For this review, take the finished solid that the model builds, in its own axes (mm). Face numbers are marked on the shaded views. A direction names the side the tool comes from. Coordinates: 2 decimals unless noted, no trailing zeros. Loops run counter-clockwise (first coordinate to the right, second up) from the corner with the lowest first, then second, coordinate; pieces in that order, holes last. Notation, with made-up numbers: (80.25, -7.75) - (104.25, -7.75) arc R37 ccw to (104.25, 28.25) - close; hole circle Ø3 at (-30, 13). An arc over 180 degrees is marked (long way). One line per item, written item: value. Start each with the question number.
1. Take a section at D-D, the plane z = 13.5. State the section outline as (x, y) points, and give its area (3 significant figures).
2. To check wall thickness, follow line 1 (X direction, y = 33.5, z = 11.5); line 2 (Y direction, x = -11, z = 14.75); line 3 (Z direction, x = -39, y = 28). State the ranges of each line that lie inside material, in increasing order. Write a range as from..to.
3. Take a section at B-B, the plane x = -17. State the section outline as (y, z) points, and give its area (3 significant figures).
4. Take a section at C-C, the plane y = 23. State the section outline as (x, z) points, and give its area (3 significant figures).
5. Insertion check: pin 1 (1.5 mm diameter, centred on y = 24, z = 20, fed in from -X); pin 2 (4 mm diameter, centred on y = 43.5, z = 14.5, fed in from +X); pin 3 (1.8 mm diameter, centred on x = 1.5, z = 12.5, fed in from +Y). Each pin has a flat end and moves straight along its axis. Give the tip position at first contact, or say it passes through.
6. The part is to be moulded in two halves that separate along X. For the marked faces 5, 6, 7 and 8, say which applies: released by +X, released by -X, zero draft, split by the parting line, or undercut.
7. For the marked faces 1, 2, 3 and 4, list the 3-axis set-ups (+Z, -Z, +X, -X, +Y, -Y) from which the entire face can be reached by the end or side of a thin tool; tool diameter is ignored.
8. Take a section at A-A, the plane z = 19.25. State the section outline as (x, y) points.
Autodesk Inventor part; units mm, degrees
ref_plane "Work Plane1" through (0, 0, 10) normal (0, 0, 1) x (1, 0, 0)
ref_plane "Work Plane3" through (-33.4299, 11.4299, 16.4) normal (0, 0, -1) x (0, 1, 0)
ref_plane "YZ Plane" through (0, 0, 0) normal (1, 0, 0) x (0, 1, 0)
ref_plane "Work Plane1" through (0, 0, 10) normal (0, 0, 1) x (1, 0, 0)
sketch "Sketch1" plane through (0, 0, 10) normal (0, 0, 1) x (1, 0, 0)
  line L0 (-4.0299, -0.3538) -> (-2.2322, 1.4439) construction
  arc A0 (-1.4439, 2.2322) -> (-2.2322, 1.4439) centre (-0.9299, 0.9299) ccw construction
  line L1 (-1.4439, 2.2322) -> (0.3538, 4.0299) construction
  line L2 (-37.8299, 42.2137) -> (-37.8299, 45.8299) construction
  line L3 (-37.8299, 45.8299) -> (-4.0299, 45.8299) construction
  line L4 (-4.0299, 45.8299) -> (-4.0299, 42.2137) construction
  line L5 (-4.0299, 4.0299) -> (0.3538, 4.0299)
  circle A1 centre (-20.9299, 20.9299) radius 17.5
  line L6 (-20.9299, 58.9723) -> (17.1124, 20.9299) construction
  line L7 (17.1124, 20.9299) -> (-20.9299, -17.1124) construction
  line L8 (-20.9299, -17.1124) -> (-58.9723, 20.9299) construction
  line L9 (-58.9723, 20.9299) -> (-20.9299, 58.9723) construction
  line L10 (-20.9299, 58.9723) -> (-20.9299, -17.1124) construction
  line L11 (17.1124, 20.9299) -> (-58.9723, 20.9299) construction
  line L12 (-20.9299, 58.9723) -> (32.8701, 58.9723) construction
  line L13 (-43.4299, 43.4299) -> (1.5701, 43.4299) construction
  line L14 (1.5701, 43.4299) -> (1.5701, -1.5701) construction
  line L15 (1.5701, -1.5701) -> (-43.4299, -1.5701) construction
  line L16 (-43.4299, -1.5701) -> (-43.4299, 43.4299) construction
  line L17 (-43.4299, 43.4299) -> (1.5701, -1.5701) construction
  line L18 (1.5701, 43.4299) -> (-43.4299, -1.5701) construction
  line L19 (-43.4299, 5.3876) -> (-43.4299, 36.4723)
  line L20 (-43.4299, 36.4723) -> (-36.4723, 43.4299)
  line L21 (-36.4723, 43.4299) -> (-5.3876, 43.4299)
  line L22 (-5.3876, 43.4299) -> (1.5701, 36.4723)
  line L23 (1.5701, 36.4723) -> (1.5701, 5.3876)
  line L24 (1.5701, 5.3876) -> (-5.3876, -1.5701)
  line L25 (-5.3876, -1.5701) -> (-36.4723, -1.5701)
  line L26 (-36.4723, -1.5701) -> (-43.4299, 5.3876)
  line L27 (-4.0299, 42.2137) -> (-37.8299, 42.2137)
  line L28 (-4.0299, -0.3538) -> (-4.0299, 4.0299)
  circle A2 centre (-20.9299, 20.9299) radius 7.0417
  point P0 (-37.8299, 4.0299)
  dimension "d18" = 53.8
  dimension "d19" = 45
  dimension "d20" = 53.8
  dimension "d21" = 45
  dimension "d22" = 45
extrude "Extrusion1" add sketch "Sketch1" along normal blind 8 contours L28 L24 L25 L26 L19 L20 L27 L22 L23 L5 | L5 L24 L28 | L27 L20 L21 L22 | A1
sketch "Sketch3" plane through (0, 0, 10) normal (0, 0, -1) x (-1, 0, 0)
  line L0 (37.8299, -0.4701) -> (37.8299, 4.0299) construction
  line L1 (4.0299, 4.0299) -> (4.0299, -0.4701) construction
  line L2 (37.8299, -0.4701) -> (37.8299, 1.1886) construction
  line L3 (4.0299, -3.9701) -> (4.0299, -0.3538) construction
  line L4 (45.8299, 4.0299) -> (42.2137, 4.0299) construction
  line L5 (-0.3538, 4.0299) -> (-3.9701, 4.0299) construction
  line L6 (-3.9701, 37.8299) -> (-0.3538, 37.8299) construction
  line L7 (4.0299, 42.2137) -> (4.0299, 45.8299) construction
  line L8 (37.8299, 45.8299) -> (37.8299, 42.2137) construction
  line L9 (42.2137, 37.8299) -> (45.8299, 37.8299) construction
  line L10 (37.8299, 37.7299) -> (45.8299, 37.7299)
  line L11 (45.8299, 37.7299) -> (45.8299, 4.1299)
  line L12 (45.8299, 4.1299) -> (37.8299, 4.1299)
  line L13 (37.8299, 4.1299) -> (37.8299, 37.7299)
  line L14 (37.7299, 4.0299) -> (4.1299, 4.0299)
  line L15 (4.1299, 4.0299) -> (4.1299, -3.9701)
  line L16 (4.1299, -3.9701) -> (37.7299, -3.9701)
  line L17 (37.7299, -3.9701) -> (37.7299, 4.0299)
  line L18 (4.0299, 4.1299) -> (-3.9701, 4.1299)
  line L19 (-3.9701, 4.1299) -> (-3.9701, 37.7299)
  line L20 (-3.9701, 37.7299) -> (4.0299, 37.7299)
  line L21 (4.0299, 37.7299) -> (4.0299, 4.1299)
  line L22 (4.1299, 37.8299) -> (37.7299, 37.8299)
  line L23 (37.7299, 37.8299) -> (37.7299, 45.8299)
  line L24 (37.7299, 45.8299) -> (4.1299, 45.8299)
  line L25 (4.1299, 45.8299) -> (4.1299, 37.8299)
  point P0 (0, 0)
  dimension "d23" = 0.1
  dimension "d24" = 0.1
  dimension "d25" = 0.1
  dimension "d26" = 0.1
  dimension "d27" = 0.1
extrude "Extrusion3" add sketch "Sketch3" against normal up to surface (8 mm away)
sketch "Sketch4" plane through (0, 0, 18) normal (0, 0, 1) x (1, 0, 0)
  line L0 (-33.4299, 35.4299) -> (-33.4299, 11.4299) construction
  line L1 (-33.4299, 11.4299) -> (-8.4299, 11.4299) construction
  line L2 (-8.4299, 11.4299) -> (-8.4299, 35.4299) construction
  line L3 (-8.4299, 35.4299) -> (-33.4299, 35.4299) construction
  circle A0 centre (-10.4299, 33.4299) radius 1.05 construction
  circle A1 centre (-10.4299, 20.9299) radius 1.05 construction
  circle A2 centre (-31.4299, 20.9299) radius 1.05 construction
  circle A3 centre (-31.4299, 33.4299) radius 1.05 construction
  line L4 (-15.4299, 29.8299) -> (-12.4299, 29.8299) construction
  line L5 (-15.4299, 31.8299) -> (-15.4299, 29.8299) construction
  line L6 (-12.4299, 31.8299) -> (-15.4299, 31.8299) construction
  line L7 (-12.4299, 29.8299) -> (-12.4299, 31.8299) construction
  line L8 (-8.4299, 35.4299) -> (-11.9299, 35.4299)
  line L9 (-11.9299, 35.4299) -> (-11.9299, 19.4299)
  line L10 (-11.9299, 19.4299) -> (-8.4299, 19.4299)
  line L11 (-8.4299, 19.4299) -> (-8.4299, 35.4299)
  line L12 (-33.4299, 35.4299) -> (-29.9299, 35.4299)
  line L13 (-29.9299, 35.4299) -> (-29.9299, 19.4299)
  line L14 (-29.9299, 19.4299) -> (-33.4299, 19.4299)
  line L15 (-33.4299, 19.4299) -> (-33.4299, 35.4299)
  line L16 (-33.4299, 35.4299) -> (-37.4299, 35.4299)
  line L17 (-37.4299, 35.4299) -> (-37.4299, 19.4299)
  line L18 (-37.4299, 19.4299) -> (-33.4299, 19.4299)
  line L19 (-33.4299, 19.4299) -> (-33.4299, 35.4299)
  line L20 (-8.4299, 35.4299) -> (-4.4299, 35.4299)
  line L21 (-4.4299, 35.4299) -> (-4.4299, 19.4299)
  line L22 (-4.4299, 19.4299) -> (-8.4299, 19.4299)
  line L23 (-8.4299, 19.4299) -> (-8.4299, 35.4299)
  point P0 (0, 0)
  dimension "d30" = 3.5
  dimension "d31" = 16
  dimension "d32" = 3.5
  dimension "d37" = 4
  dimension "d38" = 4
ref_plane "Work Plane3" through (-33.4299, 11.4299, 16.4) normal (0, 0, -1) x (0, 1, 0)
extrude "Extrusion4" add sketch "Sketch4" along normal blind 3
sketch "Sketch5" plane through (-11.9299, 35.4299, 21) normal (0, 0, 1) x (1, 0, 0)
  circle A0 centre (1.5, -14.5) radius 1.05
  circle A1 centre (1.5, -2) radius 1.05
  circle A2 centre (-19.5, -2) radius 1.05
  circle A3 centre (-19.5, -14.5) radius 1.05
  point P0 (11.9299, -35.4299)
extrude "Extrusion5" cut sketch "Sketch5" against normal through all
sketch "Skizze12" plane through (0, 0, 10) normal (0, 0, -1) x (-1, 0, 0)
  line L0 (-0.3124, 4.1299) -> (4.1299, -0.3124)
  line L1 (4.1299, -0.3124) -> (4.1299, -3.9701)
  line L2 (4.1299, -3.9701) -> (37.7299, -3.9701) construction
  line L3 (37.7299, -3.9701) -> (37.7299, -0.3124)
  line L4 (37.7299, -0.3124) -> (42.1723, 4.1299)
  line L5 (45.8299, 4.1299) -> (42.1723, 4.1299)
  line L6 (45.8299, 37.7299) -> (45.8299, 4.1299) construction
  line L7 (42.1723, 37.7299) -> (45.8299, 37.7299)
  line L8 (42.1723, 37.7299) -> (37.7299, 42.1723)
  line L9 (37.7299, 42.1723) -> (37.7299, 45.8299)
  line L10 (37.7299, 45.8299) -> (4.1299, 45.8299) construction
  line L11 (4.1299, 45.8299) -> (4.1299, 42.1723)
  line L12 (4.1299, 42.1723) -> (-0.3124, 37.7299)
  line L13 (-3.9701, 37.7299) -> (-0.3124, 37.7299)
  line L14 (-3.9701, 4.1299) -> (-3.9701, 37.7299) construction
  line L15 (-0.3124, 4.1299) -> (-3.9701, 4.1299)
  circle A0 centre (20.9299, 20.9299) radius 7.0417 construction
  line L16 (37.9299, -4.1701) -> (3.9299, -4.1701) construction
  line L17 (3.9299, -4.1701) -> (3.9299, -0.3953)
  line L18 (3.9299, -0.3953) -> (-0.3953, 3.9299)
  line L19 (-0.3953, 3.9299) -> (-4.1701, 3.9299)
  line L20 (-4.1701, 3.9299) -> (-4.1701, 37.9299) construction
  line L21 (-4.1701, 37.9299) -> (-0.3953, 37.9299)
  line L22 (-0.3953, 37.9299) -> (3.9299, 42.2551)
  line L23 (3.9299, 42.2551) -> (3.9299, 46.0299)
  line L24 (3.9299, 46.0299) -> (37.9299, 46.0299) construction
  line L25 (37.9299, 46.0299) -> (37.9299, 42.2551)
  line L26 (37.9299, 42.2551) -> (42.2551, 37.9299)
  line L27 (42.2551, 37.9299) -> (46.0299, 37.9299)
  line L28 (46.0299, 37.9299) -> (46.0299, 3.9299) construction
  line L29 (46.0299, 3.9299) -> (42.2551, 3.9299)
  line L30 (42.2551, 3.9299) -> (37.9299, -0.3953)
  line L31 (37.9299, -0.3953) -> (37.9299, -4.1701)
  line L32 (-3.9701, 37.7299) -> (-3.9701, 37.9299)
  line L33 (37.7299, 45.8299) -> (4.1299, 45.8299)
  line L34 (4.1299, 45.8299) -> (3.9299, 45.8299)
  line L35 (37.7299, 45.8299) -> (37.9299, 45.8299)
  line L36 (45.8299, 37.7299) -> (45.8299, 37.9299)
  line L37 (45.8299, 4.1299) -> (45.8299, 3.9299)
  line L38 (37.7299, -3.9701) -> (37.9299, -3.9701)
  line L39 (4.1299, -3.9701) -> (3.9299, -3.9701)
  line L40 (-3.9701, 4.1299) -> (-3.9701, 3.9299)
  point P0 (0, 0)
  dimension "d65" = 0.2
extrude "IM_offset" add sketch "Skizze12" against normal up to surface (8 mm away)
sketch "Sketch13" plane through (0, 0, 18) normal (0, 0, 1) x (1, 0, 0)
  line L0 (3.9701, 37.9299) -> (3.9701, 3.9299)
  line L1 (0.3953, 37.9299) -> (3.9701, 37.9299)
  line L2 (-3.9299, 42.2551) -> (0.3953, 37.9299)
  line L3 (-3.9299, 45.8299) -> (-3.9299, 42.2551)
  line L4 (-37.9299, 45.8299) -> (-3.9299, 45.8299)
  line L5 (-37.9299, 42.2551) -> (-37.9299, 45.8299)
  line L6 (-42.2551, 37.9299) -> (-37.9299, 42.2551)
  line L7 (-45.8299, 37.9299) -> (-42.2551, 37.9299)
  line L8 (-45.8299, 3.9299) -> (-45.8299, 37.9299)
  line L9 (-42.2551, 3.9299) -> (-45.8299, 3.9299)
  line L10 (-37.9299, -0.3953) -> (-42.2551, 3.9299)
  line L11 (-37.9299, -3.9701) -> (-37.9299, -0.3953)
  line L12 (-3.9299, -3.9701) -> (-37.9299, -3.9701)
  line L13 (-3.9299, -0.3953) -> (-3.9299, -3.9701)
  line L14 (0.3953, 3.9299) -> (-3.9299, -0.3953)
  line L15 (3.9701, 3.9299) -> (0.3953, 3.9299)
  circle A0 centre (-20.9299, 20.9299) radius 7.0417
  line L16 (-33.2963, 30.7242) -> (-29.9299, 30.7242)
  line L17 (-29.9299, 30.7242) -> (-29.9299, 35.4299)
  line L18 (-29.9299, 35.4299) -> (-37.4299, 35.4299)
  line L19 (-37.4299, 35.4299) -> (-37.4299, 19.4299)
  line L20 (-37.4299, 19.4299) -> (-29.9299, 19.4299)
  line L21 (-29.9299, 19.4299) -> (-29.9299, 22.7242)
  line L22 (-29.9299, 22.7242) -> (-33.2963, 22.7242)
  line L23 (-33.2963, 22.7242) -> (-33.2963, 30.7242)
  circle A1 centre (-31.4299, 33.4299) radius 1.05
  circle A2 centre (-31.4299, 20.9299) radius 1.05
  line L24 (-8.2963, 22.7242) -> (-11.9299, 22.7242)
  line L25 (-11.9299, 22.7242) -> (-11.9299, 19.4299)
  line L26 (-11.9299, 19.4299) -> (-4.4299, 19.4299)
  line L27 (-4.4299, 19.4299) -> (-4.4299, 35.4299)
  line L28 (-4.4299, 35.4299) -> (-11.9299, 35.4299)
  line L29 (-11.9299, 35.4299) -> (-11.9299, 30.7242)
  line L30 (-11.9299, 30.7242) -> (-8.2963, 30.7242)
  line L31 (-8.2963, 30.7242) -> (-8.2963, 22.7242)
  circle A3 centre (-10.4299, 20.9299) radius 1.05
  circle A4 centre (-10.4299, 33.4299) radius 1.05
  point P0 (0, 0)
properties part number "20_Cube_Insert_RaspiCam_v3"
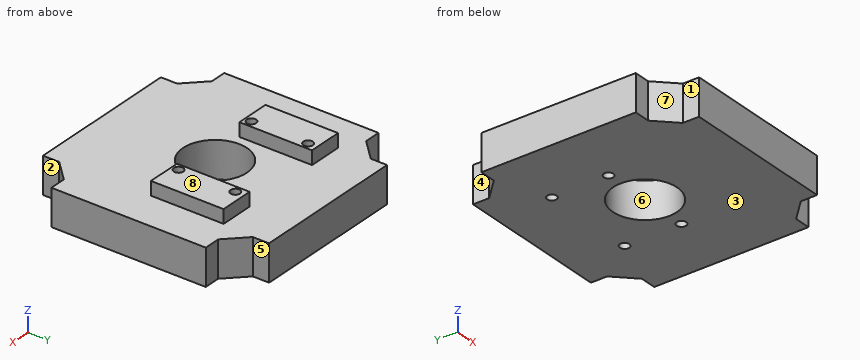
Solutions:
1. outline: (-45.83, 3.93) - (-42.26, 3.93) - (-37.93, -0.4) - (-37.93, -3.97) - (-3.93, -3.97) - (-3.93, -0.4) - (0.4, 3.93) - (3.97, 3.93) - (3.97, 37.93) - (0.4, 37.93) - (-3.93, 42.26) - (-3.93, 45.83) - (-37.93, 45.83) - (-37.93, 42.26) - (-42.26, 37.93) - (-45.83, 37.93) - close; hole circle Ø2.1 at (-31.43, 20.93); hole circle Ø2.1 at (-31.43, 33.43); hole circle Ø14.08 at (-20.93, 20.93); hole circle Ø2.1 at (-10.43, 20.93); hole circle Ø2.1 at (-10.43, 33.43)
1. area: 2,100 mm2
2. line 1: -45.83..-32.48, -30.38..-11.48, -9.38..3.97
2. line 2: -3.97..20.05, 21.81..32.55, 34.31..45.83
2. line 3: 10..18
3. outline: (-3.97, 10) - (15.09, 10) - (15.09, 18) - (-3.97, 18) - close; (26.77, 10) - (45.83, 10) - (45.83, 18) - (26.77, 18) - close
3. area: 305 mm2
4. outline: (-45.83, 10) - (-27.66, 10) - (-27.66, 18) - (-29.93, 18) - (-29.93, 21) - (-37.43, 21) - (-37.43, 18) - (-45.83, 18) - close; (-14.2, 10) - (3.97, 10) - (3.97, 18) - (-4.43, 18) - (-4.43, 21) - (-11.93, 21) - (-11.93, 18) - (-14.2, 18) - close
4. area: 336 mm2
5. pin 1: x = -37.43
5. pin 2: x = -3.17
5. pin 3: y = 37.93
6. face 5: released by +X
6. face 6: undercut
6. face 7: released by -X
6. face 8: zero draft
7. face 1: +Z, -Z, -X, -Y
7. face 2: +Z, -Z, +X, -Y
7. face 3: -Z, +X, -X, +Y, -Y
7. face 4: +Z, -Z, -X, +Y
8. outline: (-37.43, 19.43) - (-29.93, 19.43) - (-29.93, 35.43) - (-37.43, 35.43) - close; (-11.93, 19.43) - (-4.43, 19.43) - (-4.43, 35.43) - (-11.93, 35.43) - close; hole circle Ø2.1 at (-31.43, 20.93); hole circle Ø2.1 at (-31.43, 33.43); hole circle Ø2.1 at (-10.43, 20.93); hole circle Ø2.1 at (-10.43, 33.43)
